Design review of the part built by this model. Coordinates are the model's own, in mm. A direction names the side the tool comes from. Round coordinates to 2 decimals unless told otherwise and drop trailing zeros. Loops run counter-clockwise (first coordinate to the right, second up) from the corner with the lowest first, then second, coordinate; pieces in that order, holes last. Notation, with made-up numbers: M -15,58.5 L -1,58.5 A18 cw -1,71.5 Z; hole C 50.5,83 d1. An arc over 180 degrees is marked long. One line per item, written item: value. Start each with the question number.
Item 1: Clearance check with flat-ended pins moving along their axes: pin 1 (1 mm diameter, centred on y = -0.5, z = -4, fed in from -X); pin 2 (2 mm diameter, centred on y = -4.5, z = 1.5, fed in from -X); pin 3 (2 mm diameter, centred on x = 10, y = -3, fed in from +Z). State where each tip first meets the part, or that it passes through.
Item 2: We need section A-A (z = 0). State how many separate pieces and enclosed holes the cut face has, then the cut area to 3 significant figures.
Item 3: For line 1 along Z through (x, y) = (0, -0.45); line 2 along X through (y, z) = (-2.5, 5.5); line 3 along X through (y, z) = (-0.5, -6), list the stretches that pass through material, from the lowest coordinate up.
Item 4: We need section C-C (y = -3). Write out the cut boundary in (x, z).
Item 5: Mouldability with a two-part tool opening along Z and no side actions: class faces 4 (the cylindrical face through (0, -5, -7)), 5 (the flat face through (1.8, -3, -10)), 6 (the flat face through (-10, -2, 1)) as released by +Z, released by -Z, zero draft, split by the parting line, or undercut.
Item 6: For faces 1 (the flat face through (6, -5, 0)), 2 (the cylindrical face through (1.333, 0.493, -6.004)), 3 (the cylindrical face through (7.2, -3, 0)), list the 3-axis set-ups (+Z, -Z, +X, -X, +Y, -Y) from which the entire face can be reached by the end or side of a thin tool; tool diameter is ignored.
from build123d import *

# Parameters (mm, degrees)
F0_R      = 11
F1_DEPTH  = 6
F2_R      = 16
F3_DEPTH  = 2
F5_R      = 1
F6_DEPTH  = 4.001
F9_DEPTH  = 2
F10_R     = 0.3
F11_R     = 6.15
F12_DEPTH = 1
F4_R      = 2
F13_DEPTH = 7.001


with BuildPart() as f1:
    # F0 (on Front) → F1 (new body)
    with BuildSketch(Plane.XZ):
        Circle(F0_R)
    extrude(amount=F1_DEPTH)

    # F2 (on face) → F3 (cut)
    with BuildSketch(Plane.XZ.offset(6)):
        Circle(F2_R)
        with BuildLine():
            ThreePointArc((6, -3.6055512755), (0, -7), (-6, -3.6055512755))
            Line((-6, -3.6055512755), (-6, 3.6055512755))
            ThreePointArc((-6, 3.6055512755), (0, 7), (6, 3.6055512755))
            Line((6, 3.6055512755), (6, -3.6055512755))
        make_face(mode=Mode.SUBTRACT)
    extrude(amount=-F3_DEPTH, mode=Mode.SUBTRACT)

    # F5 (on face) → F6 (cut, through all)
    with BuildSketch(Plane.XZ.offset(4)):
        with Locations((0, 9)):
            Circle(F5_R)
        with Locations((-6.3639610307, 6.3639610307)):
            Circle(F5_R)
        with Locations((-9, 0)):
            Circle(F5_R)
        with Locations((-6.3639610307, -6.3639610307)):
            Circle(F5_R)
        with Locations((0, -9)):
            Circle(F5_R)
        with Locations((6.3639610307, -6.3639610307)):
            Circle(F5_R)
        with Locations((9, 0)):
            Circle(F5_R)
        with Locations((6.3639610307, 6.3639610307)):
            Circle(F5_R)
    extrude(amount=-F6_DEPTH, mode=Mode.SUBTRACT)

    # F8 (on face) → F9 (cut)
    with BuildSketch(Plane.XZ.offset(4)):
        with BuildLine():
            Line((-1.8, 11.6544359102), (-1.8, 9))
            ThreePointArc((-1.8, 9), (0, 7.2), (1.8, 9))
            Line((1.8, 9), (1.8, 11.6544359102))
            Line((1.8, 11.6544359102), (-1.8, 11.6544359102))
        make_face()
        with BuildLine():
            Line((-11.6544359102, -1.8), (-9, -1.8))
            ThreePointArc((-9, -1.8), (-7.2, 0), (-9, 1.8))
            Line((-9, 1.8), (-11.6544359102, 1.8))
            Line((-11.6544359102, 1.8), (-11.6544359102, -1.8))
        make_face()
        with BuildLine():
            Line((1.8, -11.6544359102), (1.8, -9))
            ThreePointArc((1.8, -9), (0, -7.2), (-1.8, -9))
            Line((-1.8, -9), (-1.8, -11.6544359102))
            Line((-1.8, -11.6544359102), (1.8, -11.6544359102))
        make_face()
        with BuildLine():
            Line((11.6544359102, 1.8), (9, 1.8))
            ThreePointArc((9, 1.8), (7.2, 0), (9, -1.8))
            Line((9, -1.8), (11.6544359102, -1.8))
            Line((11.6544359102, -1.8), (11.6544359102, 1.8))
        make_face()
    extrude(amount=-F9_DEPTH, mode=Mode.SUBTRACT)

    # F10
    f10_edges = [f1.edges().sort_by_distance(p)[0] for p in [
        (0, -6, -7),
        (-6, -6, 0),
        (6, -6, 0),
        (0, -6, 7),
        (7.778175, -4, -7.778175),
        (-7.778175, -4, -7.778175),
        (-7.778175, -4, 7.778175),
        (7.778175, -4, 7.778175),
    ]]
    fillet(f10_edges, radius=F10_R)

    # F11 (on face) → F12 (join)
    with BuildSketch(Plane(origin=(0, 0, 0), x_dir=(-1, 0, 0), z_dir=(0, 1, 0))):
        Circle(F11_R)
    extrude(amount=F12_DEPTH)

    # F4 (on face) → F13 (cut, through all)
    with BuildSketch(Plane.XZ.offset(6)):
        Circle(F4_R)
    extrude(amount=-F13_DEPTH, mode=Mode.SUBTRACT)


solid = f1.part
A:
1. pin 1: x = -10.43
1. pin 2: x = -10.85
1. pin 3: z = 6.32
2. separate pieces: 4
2. enclosed holes: 0
2. area: 73.1 mm2
3. line 1: -11 to -10, -8 to -2, 2 to 8, 10 to 11
3. line 2: -9.53 to -6.87, -5.86 to 5.86, 6.87 to 9.53
3. line 3: -9.22 to -7.3, -5.43 to 5.43, 7.3 to 9.22
4. outline: M -10.85,-1.8 A11 ccw -1.8,-10.85 L -1.8,-9 A1.8 cw 1.8,-9 L 1.8,-10.85 A11 ccw 10.85,-1.8 L 9,-1.8 A1.8 cw 9,1.8 L 10.85,1.8 A11 ccw 1.8,10.85 L 1.8,9 A1.8 cw -1.8,9 L -1.8,10.85 A11 ccw -10.85,1.8 L -9,1.8 A1.8 cw -9,-1.8 Z; hole C -6.36,-6.36 d2; hole C -6.36,6.36 d2; hole C 0,0 d4; hole C 6.36,-6.36 d2; hole C 6.36,6.36 d2
5. face 4: released by -Z
5. face 5: zero draft
5. face 6: undercut
6. face 1: +Z, -Z, +X, -Y
6. face 2: +Y
6. face 3: +X, -Y
